Autodesk Inventor part; units mm, degrees
ref_plane "Work Plane1" through (0, 0, 4) normal (0, 0, 1) x (1, 0, 0)
ref_plane "Work Plane3" through (0, 4, 0) normal (0, 1, 0) x (-1, 0, 0)
ref_plane "YZ Plane" through (0, 0, 0) normal (1, 0, 0) x (0, 1, 0)
sketch "Sketch1" plane through (0, 0, 0) normal (0, 0, 1) x (1, 0, 0)
  line L0 (0, 0) -> (0, 4)
  line L1 (0, 4) -> (20, 4)
  line L2 (20, 4) -> (20, 0)
  line L3 (20, 0) -> (0, 0)
  dimension "d0" = 8
  dimension "d1" = 20
revolve "Revolution1" add sketch "Sketch1" angle 360 about axis through (20, 0, 0) along (-1, 0, 0)
ref_plane "Work Plane1" through (0, 0, 4) normal (0, 0, 1) x (1, 0, 0)
ref_plane "Work Plane3" through (0, 4, 0) normal (0, 1, 0) x (-1, 0, 0)
sketch "Sketch2" plane through (0, 0, 4) normal (0, 0, 1) x (1, 0, 0)
  line L0 (0, 4) -> (0, -4)
  line L1 (20, 4) -> (20, -4)
  line L2 (20, 4) -> (0, 4)
  line L3 (20, -4) -> (0, -4)
  line L4 (0, 1.5) -> (10, 1.5)
  line L5 (10, 1.5) -> (10, -1.5)
  line L6 (10, -1.5) -> (0, -1.5)
  line L7 (0, -1.5) -> (0, 1.5)
  point P0 (0, 0)
  point P1 (10, 0)
  point P2 (0, 0)
  point P3 (0, -1.5)
  dimension "d4" = 10
  dimension "d5" = 3
extrude "Extrusion1" cut sketch "Sketch2" against normal blind 8 contours L4 L5 L6 L0
sketch "Sketch4" plane through (0, 4, 0) normal (0, 1, 0) x (-1, 0, 0)
  line L0 (0, -3.7081) -> (0, 3.7081)
  line L1 (-20, -4) -> (-20, 4)
  point P0 (0, 0)
  point P1 (-4, 0)
  point P2 (0, 0)
  dimension "d18" = 16
hole "Hole2" at (4, 4, 0) direction (0, -1, 0) diameter 4 depth 8
sketch "Sketch5" plane through (20, 0, 0) normal (1, 0, 0) x (0, 0, -1)
  circle A0 centre (0, 0) radius 4
hole "Hole3" at (20, 0, 0) direction (-1, 0, 0) diameter 4.134 depth 8
properties part number "17"
Here's how the part is built. I have some questions about the finished solid (model axes, mm). A direction names the side the tool comes from. Round coordinates to 2 decimals unless told otherwise and drop trailing zeros. Loops run counter-clockwise (first coordinate to the right, second up) from the corner with the lowest first, then second, coordinate; pieces in that order, holes last. Notation, with made-up numbers: (33, 63.25) -> (76, 63.25) arc R24 ccw to (76, 79.25) -> close; hole circle Ø1 at (-14, 64). An arc over 180 degrees is marked (long way). Write each question's results on one line, items separated by ' | '.
(1) If I drill on L1, parallel to Z at x = 18.25, y = 0; L2, parallel to X at y = 2.3, z = 0, over which ranges is the centre line in solid material (lowest first)?
Worked answers:
L1: -4 to -2.07, 2.07 to 4 | L2: 0 to 2, 6 to 20
(2) If we section it at C-C, the plane x = 7.25: List the corners of the cut face in (y, z) for me, then the cut area to 3 significant figures.
Worked answers:
outline: (-1.5, -3.71) -> (-1.5, 3.71) arc R4 ccw to start; (1.5, -3.71) arc R4 ccw to (1.5, 3.71) -> close | area: 26.8 mm2
(3) For faces 1 (the face through (15.94, 1.26, 1.64)), 2 (the face through (0, -2, 0)), 3 (the face through (10, 0, 0)), which set-ups out of +Z, -Z, +X, -X, +Y, -Y let a thin tool reach every point of the face, with its end or its side?
Worked answers:
face 1: +X | face 2: +Z, -Z, -X, +Y, -Y | face 3: +Z, -Z, -X
(4) If we section it at A-A, the plane z = 0: List the corners of the cut face in (x, y) for me.
Worked answers:
outline: (0, -4) -> (2, -4) -> (2, -1.5) -> (0, -1.5) -> close; (0, 1.5) -> (2, 1.5) -> (2, 4) -> (0, 4) -> close; (6, -4) -> (20, -4) -> (20, -2.07) -> (12, -2.07) -> (12, 2.07) -> (20, 2.07) -> (20, 4) -> (6, 4) -> (6, 1.5) -> (10, 1.5) -> (10, -1.5) -> (6, -1.5) -> close
(5) If we section it at D-D, the plane y = 3: List the corners of the cut face in (x, z) for me, then the cut area to 3 significant figures.
Worked answers:
outline: (0, -2.65) -> (20, -2.65) -> (20, 2.65) -> (0, 2.65) -> close; hole circle Ø4 at (4, 0) | area: 93.3 mm2
(6) We'd pull the mould along Z, two halves only. Please class faces 4 (the face through (6, 1.5, 1)), 5 (the face through (12, 0, 0)), 6 (the face through (10.14, 3.695, -1.532)): released by +Z, released by -Z, zero draft, split by the parting line, or undercut.
Worked answers:
face 4: zero draft | face 5: undercut | face 6: split by the parting line
(7) If we section it at B-B, the plane y = 0: List the corners of the cut face in (x, z) for me, then the cut area to 3 significant figures.
Worked answers:
outline: (10, -4) -> (20, -4) -> (20, -2.07) -> (12, -2.07) -> (12, 2.07) -> (20, 2.07) -> (20, 4) -> (10, 4) -> close | area: 46.9 mm2
(8) For P1, Ø3, axis at x = 4, z = 0, coming from the -Y side; P2, Ø1.5, axis at y = 0.5, z = 1.5, coming from the -X side; P3, Ø4, axis at x = 6, y = 0.5, coming from the -Z side, each with a flat end and sliding along its axis, tell me the tip position at first contact or that it passes through.
Worked answers:
P1: through | P2: x = 10 | P3: z = -3.71
